Can you work these out from the drawing? Everything is in mm from the part's minimum corner. Round coordinates to 2 decimals unless told otherwise and drop trailing zeros. Write each loop counter-clockwise with the first axis right and the second up, starting at its lowest first coordinate (ties: lowest second). Pieces come first, ordered by that corner, then holes. Notation, with made-up numbers: M 37,65 L 45,65 A18 ccw 45,94 Z; hole C 10,50.5 d11. An arc over 180 degrees is marked long. Use one line per item in the form item = value. Start each with the question number.
Q1. I'm going to push flat-ended pins straight in: pin 1 Ø2 at (y, z) = (81.5, 15) entering from +X; pin 2 Ø8 at (y, z) = (12.5, 14.5) entering from -X. Where does each tip first touch, or does it pass through?
Q2. I need wall thicknesses on line 1 along X through (y, z) = (34, 20.5); line 2 along X through (y, z) = (27.5, 2); line 3 along Z through (x, y) = (175, 49.5). Which ranges of each line are inside material? Lowest first, please. Write a range as from..to.
Q3. I want a section at B-B on x = 165.5. List the corners of the cut face in (y, z) for me (1 decimal), and give its area (3 significant figures).
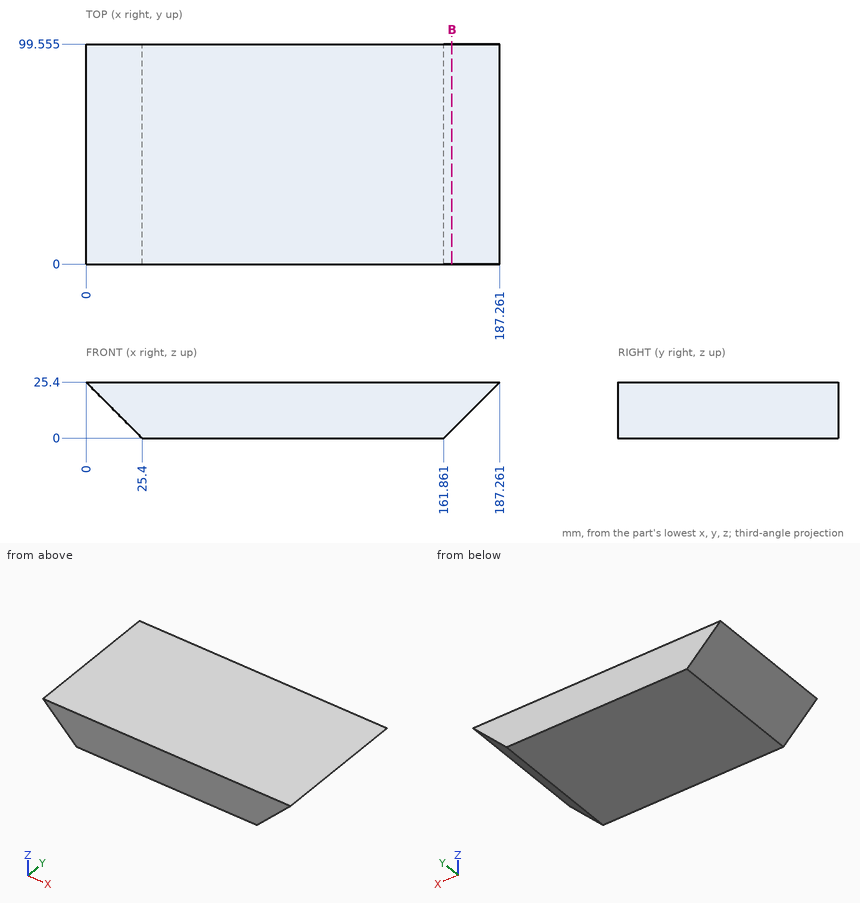
Reported:
q1.pin_1 = 177.86
q1.pin_2 = 6.9
q2.line_1 = 4.9..182.36
q2.line_2 = 23.4..163.86
q2.line_3 = 13.14..25.4
q3.outline = M 0,3.6 L 99.6,3.6 L 99.6,25.4 L 0,25.4 Z
q3.area = 2,170 mm^2
